Build history of the part. All positions in model axes, mm. A direction names the side the tool comes from. Give positions to 0.01 mm unless a question says otherwise; leave off trailing zeros. Write each loop counter-clockwise with the first axis right and the second up, starting at its lowest first coordinate (ties: lowest second). Pieces come first, ordered by that corner, then holes. Notation, with made-up numbers: M -20.75,-13 L 3.25,-13 A31 cw 3.25,18 Z; hole C 49,80 d5. An arc over 180 degrees is marked long. Return JSON: item names as keys, results as strings. Group by question number.
Q1. Wall check: probe 1 along Y at (x, z) = (0, 129); probe 2 along X at (y, z) = (0.5, 49.5). Give the ranges that are in metal, low to high.
Q2. Pull direction X, two halves, no side cores. Call faces 1 (the flat face through (2, -2, 136)), 2 (the flat face through (0, 0, 116)), 3 (the cylindrical face through (-1.08, -4.88, 66.8)): +X half, -X half, draft (parallel to the pull), parting line (faces both ways), or undercut.
Q3. Band-saw the part on A-A, the plane y = 0. Give the cut face in (x, z).
Q4. Band-saw the part on C-C, the plane z = 54.5. Give the cut face in (x, y).
Q5. Flat gauge pins, fed straight in: pin 1 Ø3.5 at (x, y) = (0, 0) entering from +Z; pin 2 Ø3 at (x, z) = (4, 28.5) entering from -Y; pin 3 Ø2 at (x, z) = (2, 14) entering from +Y. Where does each tip first touch, or does it go through?
Q6. Tool access for faces 4 (the flat face through (0, 0, 0)), 5 (the cylindrical face through (0, -2, 126)): list every direction of +Z, -Z, +X, -X, +Y, -Y with a clear straight run to the whole face (end or side of a thin tool).
from build123d import *

# Parameters (mm, degrees)
SKETCH1_R           = 5
BOSS_EXTRUDE1_DEPTH = 136
SKETCH2_R           = 2
CUT_EXTRUDE1_DEPTH  = 20
FILLET1_R           = 0.5
FILLET2_R           = 0.5


with BuildPart() as part:
    # Sketch1 → Boss-Extrude1 (new body)
    with BuildSketch(Plane.XY):
        Circle(SKETCH1_R)
    extrude(amount=BOSS_EXTRUDE1_DEPTH)

    # Sketch2 → Cut-Extrude1 (cut)
    with BuildSketch(Plane.XY.offset(136)):
        Circle(SKETCH2_R)
    extrude(amount=-CUT_EXTRUDE1_DEPTH, mode=Mode.SUBTRACT)

    # Fillet1
    fillet1_edges = [part.edges().sort_by_distance(p)[0] for p in [
        (-5, 0, 136),
    ]]
    fillet(fillet1_edges, radius=FILLET1_R)

    # Fillet2
    fillet2_edges = [part.edges().sort_by_distance(p)[0] for p in [
        (-2, 0, 136),
    ]]
    fillet(fillet2_edges, radius=FILLET2_R)


solid = part.part
From the geometry:
{
 "1": {"probe 1": "y = -5 to -2, 2 to 5", "probe 2": "x = -4.97 to 4.97"},
 "2": {"face 1": "draft", "face 2": "undercut", "face 3": "parting line"},
 "3": {"outline": "M -5,0 L 5,0 L 5,135.5 A0.5 ccw 4.5,136 L 2.5,136 A0.5 ccw 2,135.5 L 2,116 L -2,116 L -2,135.5 A0.5 ccw -2.5,136 L -4.5,136 A0.5 ccw -5,135.5 Z"},
 "4": {"outline": "C 0,0 d10"},
 "5": {"pin 1": "stops at z = 116", "pin 2": "stops at y = -4.33", "pin 3": "stops at y = 4.9"},
 "6": {"face 4": "-Z, +X, -X, +Y, -Y", "face 5": "+Z"}
}
